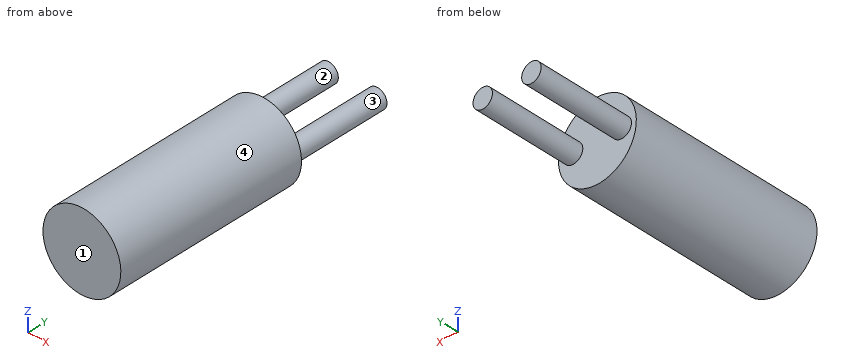
```python
from build123d import *

# Parameters (mm, degrees)
SKETCH_1_R      = 4
EXTRUDE_1_DEPTH = 20
SKETCH_2_R      = 1
EXTRUDE_2_DEPTH = 10


with BuildPart() as part:
    # 草图1 → 凸台-拉伸1 (new body)
    with BuildSketch(Plane(origin=(0, 0, 0), x_dir=(1, 0, 0), z_dir=(0, 1, 0))):
        with Locations(Location((0, 0, 0), (0, 0, 270))):
            Circle(SKETCH_1_R)
    extrude(amount=EXTRUDE_1_DEPTH)

    # 草图2 → 凸台-拉伸2 (add)
    with BuildSketch(Plane(origin=(0, 20, 0), x_dir=(1, 0, 0), z_dir=(0, 1, 0))):
        with Locations(Location((-2.5, 0, 0), (0, 0, 270))):
            Circle(SKETCH_2_R)
    extrude_2 = extrude(amount=EXTRUDE_2_DEPTH)

    # 镜向1: 凸台-拉伸2 across plane
    add(extrude_2.mirror(Plane(origin=(0, 0, 0), x_dir=(0, 0, 1), z_dir=(1, 0, 0))))


solid = part.part
```
Read the model definition and answer for the solid it produces. Units are mm, in the model's axes. Face numbers are marked on the shaded views. Coordinates: 2 decimals unless noted, no trailing zeros. Loops run counter-clockwise (first coordinate to the right, second up) from the corner with the lowest first, then second, coordinate; pieces in that order, holes last. Notation, with made-up numbers: (-2, 1.5) - (38, 1.5) arc R15 cw to (38, 17.5) - close; hole circle Ø11 at (-39.75, 29). An arc over 180 degrees is marked (long way). Answer in a Markdown table with one row per item.
1. Straight lines are drawn through the part: line 1 (X direction, y = 24.5, z = 0); line 2 (Y direction, x = 0.25, z = 1); line 3 (Z direction, x = 1.75, y = 28.25). For each, find the intervals that lie inside material, in ascending order.
Conclusion:
| item | result |
|---|---|
| line 1 | x = -3.5 to -1.5, 1.5 to 3.5 |
| line 2 | y = 0 to 20 |
| line 3 | z = -0.66 to 0.66 |
2. Determine the mould class of the marked faces 1, 2, 3 and 4 for opening direction X: +X half, -X half, draft (parallel to the pull), parting line (faces both ways), or undercut.
Conclusion:
| item | result |
|---|---|
| face 1 | draft |
| face 2 | undercut |
| face 3 | undercut |
| face 4 | parting line |
3. Find section B-B, the plane y = 24. Write down the section's boundary in (x, z), then the cut area to 3 significant figures.
Conclusion:
| item | result |
|---|---|
| outline | circle Ø2 at (-2.5, 0); circle Ø2 at (2.5, 0) |
| area | 6.28 mm² |
4. Find section D-D, the plane x = -2. Write down the section's boundary in (y, z).
Conclusion:
| item | result |
|---|---|
| outline | (0, -3.46) - (20, -3.46) - (20, -0.87) - (30, -0.87) - (30, 0.87) - (20, 0.87) - (20, 3.46) - (0, 3.46) - close |
5. Find section A-A, the plane z = 0. Write down the section's boundary in (x, y), then the cut area to 3 significant figures.
Conclusion:
| item | result |
|---|---|
| outline | (-4, 0) - (4, 0) - (4, 20) - (3.5, 20) - (3.5, 30) - (1.5, 30) - (1.5, 20) - (-1.5, 20) - (-1.5, 30) - (-3.5, 30) - (-3.5, 20) - (-4, 20) - close |
| area | 200 mm² |
6. Find section C-C, the plane y = 2.75. Write down the section's boundary in (x, z), then the cut area to 3 significant figures.
Conclusion:
| item | result |
|---|---|
| outline | circle Ø8 at (0, 0) |
| area | 50.3 mm² |
